Job drawing, mm, ordinate dimensions from the low corner. One solid piece. Give positions to 0.01 mm unless a question says otherwise; leave off trailing zeros. Loops run counter-clockwise (first coordinate to the right, second up) from the corner with the lowest first, then second, coordinate; pieces in that order, holes last. Notation, with made-up numbers: (-37.5, -22) - (-24.5, -22) arc R25 ccw to (-24.5, 3) - close; hole circle Ø11 at (38.5, 39.25). An arc over 180 degrees is marked (long way). Use a Markdown table: item, result.
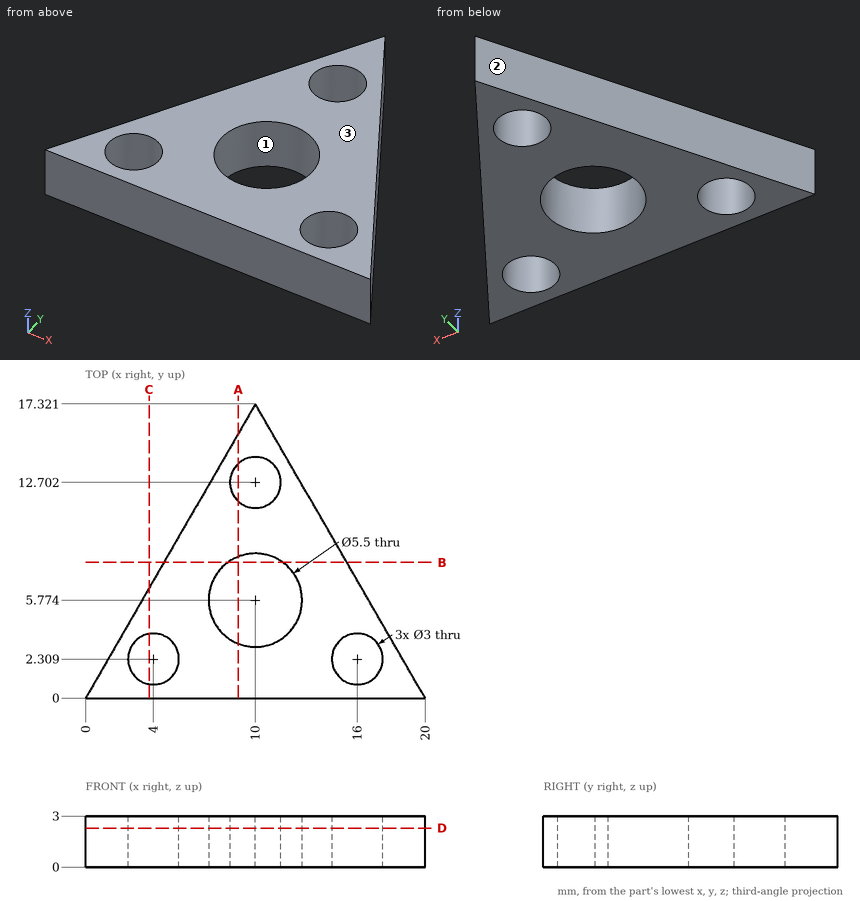
(1) Slice it at B-B, the plane y = 8. Write the cut outline in (x, z) (1 decimal), plus the area to 3 significant figures.
Computed:
| item | result |
|---|---|
| outline | (4.6, 0) - (8.4, 0) - (8.4, 3) - (4.6, 3) - close; (11.6, 0) - (15.4, 0) - (15.4, 3) - (11.6, 3) - close |
| area | 22.6 mm² |
(2) Mould opens along X. For the marked faces 1, 2 and 3 say: pulls with the +X half, pulls with the -X half, needs draft (parallel to the pull), parting line crosses it, or undercut.
Computed:
| item | result |
|---|---|
| face 1 | undercut |
| face 2 | pulls with the -X half |
| face 3 | needs draft |
(3) Slice it at C-C, the plane x = 3.75. Write the cut outline in (y, z) (1 decimal).
Computed:
| item | result |
|---|---|
| outline | (0, 0) - (0.8, 0) - (0.8, 3) - (0, 3) - close; (3.8, 0) - (6.5, 0) - (6.5, 3) - (3.8, 3) - close |
(4) Slice it at A-A, the plane x = 9. Write the cut outline in (y, z) (1 decimal).
Computed:
| item | result |
|---|---|
| outline | (0, 0) - (3.2, 0) - (3.2, 3) - (0, 3) - close; (8.3, 0) - (11.6, 0) - (11.6, 3) - (8.3, 3) - close; (13.8, 0) - (15.6, 0) - (15.6, 3) - (13.8, 3) - close |
(5) Slice it at D-D, the plane z = 2.3. Write the cut outline in (x, y), plus the area to 3 significant figures.
Computed:
| item | result |
|---|---|
| outline | (0, 0) - (20, 0) - (10, 17.32) - close; hole circle Ø3 at (4, 2.31); hole circle Ø5.5 at (10, 5.77); hole circle Ø3 at (10, 12.7); hole circle Ø3 at (16, 2.31) |
| area | 128 mm² |
(6) Pin check, flat tips, straight feed: P1, Ø5, axis at x = 10, y = 5.77, coming from the +Z side; P2, Ø1.5, axis at y = 2.5, z = 1, coming from the +X side. Stop position of each tip, or through.
Computed:
| item | result |
|---|---|
| P1 | through |
| P2 | x = 18.99 |
(7) Drill centre lines: probe 1 along X at (y, z) = (1, 2.4) (1 decimal); probe 2 along X at (y, z) = (13.5, 0.8) (1 decimal); probe 3 along X at (y, z) = (7.5, 1.95). Where is each one in solid material? Low to high. Write a range as [from, to].
Computed:
| item | result |
|---|---|
| probe 1 | [0.6, 3.3], [4.7, 15.3], [16.7, 19.4] |
| probe 2 | [7.8, 8.7], [11.3, 12.2] |
| probe 3 | [4.33, 7.86], [12.14, 15.67] |
